from build123d import *

# Parameters (mm, degrees)
CROQUIS1_R                 = 30.5
SALIENTE_EXTRUIR1_DEPTH    = 3
CROQUIS2_R                 = 2
CORTAR_EXTRUIR1_DEPTH      = 4
CORTAR_EXTRUIR3_START      = -4
CORTAR_EXTRUIR3_DEPTH      = 4
CORTAR_EXTRUIR5_START      = -4
CORTAR_EXTRUIR5_DEPTH      = 4
CORTAR_EXTRUIR6_DEPTH      = 10
CROQUIS10_R                = 2.5
CORTAR_EXTRUIR7_DEPTH      = 3
CORTAR_EXTRUIR8_DEPTH      = 44.237715166
CORTAR_EXTRUIR8_DEPTH_BACK = 44.237715166
CORTAR_EXTRUIR9_START      = -10
CORTAR_EXTRUIR9_DEPTH      = 10


with BuildPart() as part:
    # Croquis1 → Saliente-Extruir1 (new body)
    with BuildSketch(Plane(origin=(0, 0, 0), x_dir=(1, 0, 0), z_dir=(0, 1, 0))):
        with Locations(Location((0, 0, 0), (0, 0, 270))):
            Circle(CROQUIS1_R)
    extrude(amount=SALIENTE_EXTRUIR1_DEPTH)

    # Croquis2 → Cortar-Extruir1 (cut)
    with BuildSketch(Plane(origin=(0, 3, 0), x_dir=(1, 0, 0), z_dir=(0, 1, 0))):
        with Locations(Location((0, 0, 0), (0, 0, 270))):
            Circle(CROQUIS2_R)
    extrude(amount=-CORTAR_EXTRUIR1_DEPTH, mode=Mode.SUBTRACT)

    # Croquis5 → Cortar-Extruir3 (cut)
    with BuildSketch(Plane(origin=(0, 3, 0), x_dir=(1, 0, 0), z_dir=(0, 1, 0)).offset(CORTAR_EXTRUIR3_START)):
        with BuildLine():
            Line((28.814059068, 5), (30.087372767, 5))
            ThreePointArc((30.087372767, 5), (29.556634924, 7.526973624), (28.814059068, 10))
            Line((28.814059068, 10), (24.814059068, 10))
            Line((24.814059068, 10), (24.814059068, 5))
            Line((24.814059068, 5), (28.814059068, 5))
        make_face()
        with BuildLine():
            Line((30.087372767, -5), (28.814059068, -5))
            Line((28.814059068, -5), (24.814059068, -5))
            Line((24.814059068, -5), (24.814059068, -10))
            Line((24.814059068, -10), (28.814059068, -10))
            ThreePointArc((28.814059068, -10), (29.556634924, -7.526973624), (30.087372767, -5))
        make_face()
        with BuildLine():
            Line((-24.814059068, 5), (-24.814059068, 10))
            Line((-24.814059068, 10), (-28.814059068, 10))
            ThreePointArc((-28.814059068, 10), (-29.556634924, 7.526973624), (-30.087372767, 5))
            Line((-30.087372767, 5), (-28.814059068, 5))
            Line((-28.814059068, 5), (-24.814059068, 5))
        make_face()
        with BuildLine():
            Line((-28.814059068, -10), (-24.814059068, -10))
            Line((-24.814059068, -10), (-24.814059068, -5))
            Line((-24.814059068, -5), (-28.814059068, -5))
            Line((-28.814059068, -5), (-30.087372767, -5))
            ThreePointArc((-30.087372767, -5), (-29.556634924, -7.526973624), (-28.814059068, -10))
        make_face()
    extrude(amount=CORTAR_EXTRUIR3_DEPTH, mode=Mode.SUBTRACT)

    # Croquis7 → Cortar-Extruir5 (cut)
    with BuildSketch(Plane(origin=(0, 3, 0), x_dir=(1, 0, 0), z_dir=(0, 1, 0)).offset(CORTAR_EXTRUIR5_START)):
        Polygon((1.428390211, 22.411430151), (-0.869743118, 20.483067322), (2.34419493, 16.652845106), (4.642328259, 18.581207935), align=None)
        with BuildLine():
            Line((-24.814059068, -10), (-28.814059068, -10))
            ThreePointArc((-28.814059068, -10), (0, -30.5), (28.814059068, -10))
            Line((28.814059068, -10), (24.814059068, -10))
            add(Edge.make_bspline(
                [(24.814059068, -10), (22.863263717, -9.657344338), (20.984021298, -8.980450277), (19.168992989, -8.065339906)],
                knots=[0, 0, 0, 0, 0.087850084, 0.087850084, 0.087850084, 0.087850084], degree=3))
            Line((19.168992989, -8.065339906), (11.455541673, 1.127193412))
            Line((11.455541673, 1.127193412), (9.248678515, -0.72458465))
            add(Edge.make_bspline(
                [(9.248678515, -0.72458465), (4.033234859, 4.116641048), (-0.646914404, 9.508508747), (-5.04935939, 12.080675515)],
                knots=[0.258799312, 0.258799312, 0.258799312, 0.258799312, 0.546435258, 0.546435258, 0.546435258, 0.546435258], degree=3))
            Line((-5.04935939, 12.080675515), (-0.757422911, 15.682037831))
            Line((-0.757422911, 15.682037831), (-7.828086618, 24.108526705))
            Line((-7.828086618, 24.108526705), (-17.020619935, 16.395075389))
            Line((-17.020619935, 16.395075389), (-13.66601447, 12.397212273))
            add(Edge.make_bspline(
                [(-13.66601447, 12.397212273), (-17.403465693, 9.897923685), (-21.056529869, 3.255841362), (-24.814059068, -10)],
                knots=[0.740637404, 0.740637404, 0.740637404, 0.740637404, 1, 1, 1, 1], degree=3))
        make_face()
        Polygon((14.685884661, 6.611763511), (12.387751331, 4.683400682), (15.60168938, 0.853178467), (17.899822709, 2.781541296), align=None)
    extrude(amount=CORTAR_EXTRUIR5_DEPTH, mode=Mode.SUBTRACT)

    # Croquis9 → Cortar-Extruir6 (cut)
    with BuildSketch(Plane(origin=(0, 3, 0), x_dir=(1, 0, 0), z_dir=(0, 1, 0))):
        Polygon((7.971418181, 14.613753061), (5.673284852, 12.685390231), (8.887222901, 8.855168016), (11.18535623, 10.783530845), align=None)
    extrude(amount=-CORTAR_EXTRUIR6_DEPTH, mode=Mode.SUBTRACT)

    # Croquis10 → Cortar-Extruir7 (cut)
    with BuildSketch(Plane(origin=(0, 3, 0), x_dir=(1, 0, 0), z_dir=(0, 1, 0))):
        with Locations(Location((12, 16, 0), (0, 0, 270))):
            Circle(CROQUIS10_R)
    extrude(amount=-CORTAR_EXTRUIR7_DEPTH, mode=Mode.SUBTRACT)

    # Croquis11 → Cortar-Extruir8 (cut, two sides: drawn at the far end of the back side and taken through both)
    with BuildSketch(Plane(origin=(0, 3, 0), x_dir=(1, 0, 0), z_dir=(0, 1, 0)).offset(-CORTAR_EXTRUIR8_DEPTH_BACK)):
        with BuildLine():
            Line((30.087372767, 5), (27.814059068, 5))
            Line((27.814059068, 5), (27.814059068, -5))
            Line((27.814059068, -5), (30.087372767, -5))
            ThreePointArc((30.087372767, -5), (30.5, 0), (30.087372767, 5))
        make_face()
        with BuildLine():
            ThreePointArc((28.814059068, 10), (28.341972277, 11.268655974), (27.814059068, 12.515115586))
            Line((27.814059068, 12.515115586), (27.814059068, 10))
            Line((27.814059068, 10), (28.814059068, 10))
        make_face()
        with BuildLine():
            Line((-27.814059068, -5), (-27.814059068, 5))
            Line((-27.814059068, 5), (-30.087372767, 5))
            ThreePointArc((-30.087372767, 5), (-30.5, 0), (-30.087372767, -5))
            Line((-30.087372767, -5), (-27.814059068, -5))
        make_face()
        with BuildLine():
            Line((-28.814059068, 10), (-27.814059068, 10))
            Line((-27.814059068, 10), (-27.814059068, 12.515115586))
            ThreePointArc((-27.814059068, 12.515115586), (-28.341972277, 11.268655974), (-28.814059068, 10))
        make_face()
    extrude(amount=CORTAR_EXTRUIR8_DEPTH + CORTAR_EXTRUIR8_DEPTH_BACK, mode=Mode.SUBTRACT)

    # Croquis12 → Cortar-Extruir9 (cut)
    with BuildSketch(Plane(origin=(0, 3, 0), x_dir=(1, 0, 0), z_dir=(0, 1, 0)).offset(CORTAR_EXTRUIR9_START)):
        with BuildLine():
            Line((-0.28585192, 30.498660441), (27.814059068, 11.545031156))
            Line((27.814059068, 11.545031156), (27.814059068, 12.515115586))
            ThreePointArc((27.814059068, 12.515115586), (16.440879495, 25.689442995), (-0.28585192, 30.498660441))
        make_face()
    extrude(amount=CORTAR_EXTRUIR9_DEPTH, mode=Mode.SUBTRACT)


solid = part.part
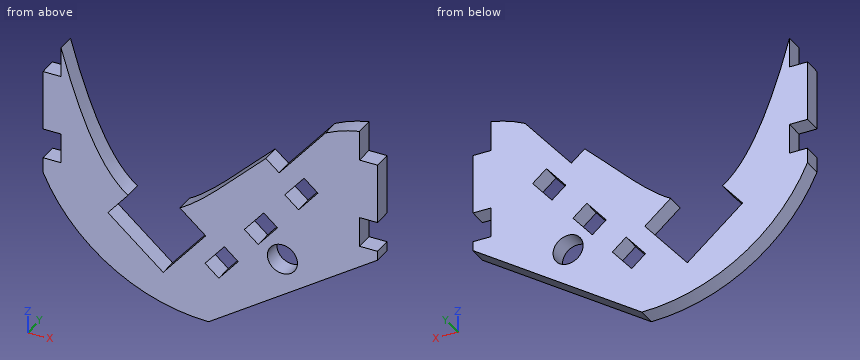
Source: CAD feature listing. Evaluate the final solid. Frame: model axes, mm. Give positions to 0.01 mm unless a question says otherwise; leave off trailing zeros. Write each loop counter-clockwise with the first axis right and the second up, starting at its lowest first coordinate (ties: lowest second). Pieces come first, ordered by that corner, then holes. Notation, with made-up numbers: (60, 41.5) -> (94, 41.5) arc R21 cw to (94, 60.5) -> close; hole circle Ø3 at (59.25, -11). An arc over 180 degrees is marked (long way). Return JSON: item names as keys, results as strings. Group by question number.
1. Section A-A, the plane z = -17.5. Output: boundary loops of the cut face in (x, y), then the cut area to 3 significant figures.
2. Material intervals for line 1 (X direction, y = 1.9, z = -16); line 2 (X direction, y = 2.55, z = -3.5); line 3 (X direction, y = 1.75, z = -1), sorted ascending. Write a range as from..to.
3. Section B-B, the plane y = 0.7. Count the separate pieces of the cut face and the enclosed holes in it, then the cut area to 3 significant figures.
4. Section D-D, the plane x = -13. Output: boundary loops of the cut face in (y, z).
5. Pin query (flat end, axial travel): pin 1 Ø0.9 at (y, z) = (1, -6.5) entering from -X; pin 2 Ø1.5 at (x, y) = (-6.5, 1.5) entering from -Z; pin 3 Ø3 at (x, z) = (16, 1) entering from -Y; pin 4 Ø1 at (x, y) = (-5, 1.5) entering from +Z. Return the tip coordinate at first contact, or that it passes through.
Determined:
{
 "1": {"outline": "(-24.98, 0) -> (-15.7, 0) -> (-15.7, 3) -> (-24.98, 3) -> close; (-2.28, 0) -> (1.63, 0) -> (1.63, 3) -> (-2.28, 3) -> close; (3.35, 0) -> (10, 0) -> (10, 3) -> (3.35, 3) -> close; (14, 0) -> (18.99, 0) -> (18.99, 3) -> (14, 3) -> close", "area": "74.5 mm2"},
 "2": {"line 1": "x = -25.97..-16.69, -1.02..9.5, 14.5..21.21", "line 2": "x = -27.81..-20.07, 4.88..13.38, 17.3..27.81", "line 3": "x = -27.81..-21.14, 7.43..11.3, 11.56..15.48, 15.78..27.81"},
 "3": {"separate pieces": "1", "enclosed holes": "4", "area": "955 mm2"},
 "4": {"outline": "(0, -27.59) -> (3, -27.59) -> (3, -19.77) -> (0, -19.77) -> close"},
 "5": {"pin 1": "stops at x = -24.81", "pin 2": "stops at z = -29.95", "pin 3": "stops at y = 0", "pin 4": "stops at z = -11.75"}
}
